Read the model definition and answer for the solid it produces. Units are mm, in the model's axes. A direction names the side the tool comes from. Give positions to 0.01 mm unless a question says otherwise; leave off trailing zeros. Loops run counter-clockwise (first coordinate to the right, second up) from the corner with the lowest first, then second, coordinate; pieces in that order, holes last. Notation, with made-up numbers: (76.5, 19) -> (98.5, 19) arc R10 ccw to (98.5, 27) -> close; hole circle Ø3 at (84.25, -34). An arc over 180 degrees is marked (long way). Return JSON: item names as keys, results as strings. Group by question number.
from build123d import *

# Parameters (mm, degrees)
EXTRUDE_2_DEPTH     = 2
CUT_EXTRUDE_2_DEPTH = 0.8
FILLET_1_R          = 0.8
SKETCH_6_W          = 43
SKETCH_6_H          = 2
SKETCH_6_H_2        = 1.9999999999999947
EXTRUDE_3_DEPTH     = 4
SKETCH_7_W          = 43
SKETCH_7_H          = 6.999999999999998
EXTRUDE_4_DEPTH     = 2
CUT_EXTRUDE_3_DEPTH = 35.3874977280988
CUT_EXTRUDE_5_DEPTH = 6
FILLET_2_R          = 4
FILLET_3_R          = 4
FILLET_4_R          = 4


# Some blends are built 0.0001 mm under size
with BuildPart() as part:
    # 草图4 → 凸台-拉伸2 (new body)
    with BuildSketch(Plane(origin=(0, 0, 0), x_dir=(1, 0, 0), z_dir=(0, 1, 0))):
        Polygon((24.499999999999996, -12.499999999999993), (24.499999999999996, 10.5), (24.499999999999996, 12.5), (-24.500000000000004, 12.5), (-28.500000000000004, 12.5), (-28.500000000000004, -12.499999999999993), (-24.500000000000004, -12.499999999999993), align=None)
        Polygon((-20.500000000000004, 10.500000000000002), (20.499999999999996, 10.5), (20.500000000000004, -10.5), (-20.5, -10.499999999999998), align=None, mode=Mode.SUBTRACT)
    extrude(amount=EXTRUDE_2_DEPTH)

    # 草图5 → 切除-拉伸2 (cut)
    with BuildSketch(Plane(origin=(0, 2, 0), x_dir=(1, 0, 0), z_dir=(0, 1, 0))):
        with BuildLine():
            Line((-24.000000000000004, 1.7499999999999991), (-24.000000000000004, 4.75))
            Line((-24.000000000000004, 4.75), (-21.000000000000004, 4.75))
            ThreePointArc((-21.000000000000004, 4.75), (-26.121320343559606, 6.871320343559683), (-24.000000000000117, 1.7499999999999991))
        make_face()
        with BuildLine():
            Line((-21.000000000000004, 4.75), (-24.000000000000004, 4.75))
            Line((-24.000000000000004, 4.75), (-24.000000000000004, 1.7499999999999991))
            ThreePointArc((-24.000000000000117, 1.7499999999999991), (-21.8786796564404, 2.6286796564403168), (-21.000000000000004, 4.749999999999999))
        make_face()
        with BuildLine():
            ThreePointArc((-21.000000000000007, -4.75), (-21.8786796564404, -2.6286796564403203), (-24.000000000000114, -1.7500000000000027))
            Line((-24.000000000000004, -1.7500000000000027), (-24.000000000000004, -4.75))
            Line((-24.000000000000004, -4.75), (-21.000000000000007, -4.75))
        make_face()
        with BuildLine():
            Line((-24.000000000000004, -4.75), (-24.000000000000004, -1.7500000000000027))
            ThreePointArc((-24.000000000000114, -1.7500000000000027), (-26.121320343559606, -6.871320343559679), (-21.000000000000007, -4.750000000000001))
            Line((-21.000000000000007, -4.75), (-24.000000000000004, -4.75))
        make_face()
        with BuildLine():
            Line((23.999999999999996, 4.75), (20.999999999999996, 4.75))
            ThreePointArc((21, 4.75), (21.878679656440315, 2.628679656440399), (23.999999999999883, 1.7500000000000027))
            Line((23.999999999999996, 1.7500000000000027), (23.999999999999996, 4.75))
        make_face()
        with BuildLine():
            ThreePointArc((24.50000000000003, 7.7080398915498), (22.063508326896304, 7.041287847477928), (21, 4.75))
            Line((20.999999999999996, 4.75), (23.999999999999996, 4.75))
            Line((23.999999999999996, 4.75), (23.999999999999996, 1.7500000000000027))
            ThreePointArc((23.999999999999883, 1.7500000000000027), (24.250878780839006, 1.760508431635119), (24.500000000000025, 1.7919601084501995))
            Line((24.499999999999996, 1.7919601084502048), (24.499999999999996, 7.708039891549795))
        make_face()
        with BuildLine():
            ThreePointArc((24.500000000000025, -1.7919601084501955), (24.25087878083901, -1.7605084316351154), (23.99999999999989, -1.7499999999999991))
            Line((24, -1.7499999999999991), (24, -4.75))
            Line((23.999999999999996, -4.75), (20.999999999999996, -4.75))
            ThreePointArc((21, -4.75), (22.0635083268963, -7.041287847477928), (24.50000000000002, -7.708039891549806))
            Line((24.499999999999996, -7.7080398915498005), (24.499999999999996, -1.7919601084501995))
        make_face()
        with BuildLine():
            Line((24, -4.75), (24, -1.7499999999999991))
            ThreePointArc((23.99999999999989, -1.7499999999999991), (21.87867965644032, -2.6286796564403963), (21, -4.75))
            Line((20.999999999999996, -4.75), (23.999999999999996, -4.75))
        make_face()
    extrude(amount=-CUT_EXTRUDE_2_DEPTH, mode=Mode.SUBTRACT)

    # 圆角1
    fillet_1_edges = [part.edges().sort_by_distance(p)[0] for p in [
        (21.000000000000117, 1.2, 4.749999999999868),
        (21, 1.2, -4.75),
        (-26.999999999999993, 1.2, 4.749999999999993),
        (-23.99999999999989, 1.2, -7.749999999999999),
    ]]
    fillet(fillet_1_edges, radius=FILLET_1_R - 0.0001)  # a hair under: the kernel refuses the full size

    # 草图6 → 凸台-拉伸3 (add)
    with BuildSketch(Plane(origin=(0, 2, 0), x_dir=(1, 0, 0), z_dir=(0, 1, 0))):
        with Locations((0.9999999999999947, 11.500000000000002)):
            Rectangle(SKETCH_6_W, SKETCH_6_H)
        with Locations((0.9999999999999982, -11.499999999999996)):
            Rectangle(SKETCH_6_W, SKETCH_6_H_2)
    extrude(amount=EXTRUDE_3_DEPTH)

    # 草图7 → 凸台-拉伸4 (add)
    with BuildSketch(Plane(origin=(0, 6, 0), x_dir=(1, 0, 0), z_dir=(0, 1, 0))):
        with Locations((0.9999999999999947, 14)):
            Rectangle(SKETCH_7_W, SKETCH_7_H)
        with Locations((0.9999999999999982, -13.999999999999996)):
            Rectangle(SKETCH_7_W, SKETCH_7_H)
    extrude(amount=EXTRUDE_4_DEPTH)

    # 草图8 → 切除-拉伸3 (cut, through all)
    with BuildSketch(Plane.XZ):
        with BuildLine():
            ThreePointArc((-10.5, -11.54), (-12.5, -13.54), (-10.5, -15.54))
            Line((-10.5, -15.54), (-6.500000000000001, -15.54))
            ThreePointArc((-6.500000000000001, -15.54), (-4.500000000000001, -13.54), (-6.500000000000001, -11.54))
            Line((-6.500000000000001, -11.54), (-10.5, -11.54))
        make_face()
        with BuildLine():
            ThreePointArc((14.5, -11.54), (12.5, -13.54), (14.5, -15.54))
            Line((14.5, -15.54), (18.500000000000004, -15.54))
            ThreePointArc((18.500000000000004, -15.54), (20.500000000000004, -13.54), (18.500000000000004, -11.54))
            Line((18.500000000000004, -11.54), (14.5, -11.54))
        make_face()
        with BuildLine():
            Line((-10.500000000000096, 11.54), (-6.500000000000095, 11.54))
            ThreePointArc((-6.500000000000095, 11.54), (-4.500000000000095, 13.54), (-6.500000000000095, 15.54))
            Line((-6.500000000000095, 15.54), (-10.500000000000096, 15.54))
            ThreePointArc((-10.500000000000096, 15.54), (-12.500000000000096, 13.54), (-10.500000000000096, 11.54))
        make_face()
        with BuildLine():
            Line((14.499999999999908, 11.54), (18.499999999999904, 11.54))
            ThreePointArc((18.499999999999904, 11.540000000000001), (20.499999999999904, 13.540000000000001), (18.499999999999904, 15.540000000000001))
            Line((18.499999999999904, 15.54), (14.499999999999908, 15.54))
            ThreePointArc((14.499999999999908, 15.54), (12.499999999999908, 13.54), (14.499999999999908, 11.54))
        make_face()
    extrude(amount=-CUT_EXTRUDE_3_DEPTH, mode=Mode.SUBTRACT)

    # 草图9 → 切除-拉伸5 (cut)
    with BuildSketch(Plane.XZ):
        with BuildLine():
            Line((14.5, -10.540000000000001), (18.500000000000004, -10.54))
            ThreePointArc((18.500000000000004, -10.54), (21.500000000000004, -13.54), (18.500000000000004, -16.54))
            Line((18.500000000000004, -16.54), (14.5, -16.54))
            ThreePointArc((14.5, -16.54), (11.500000000000002, -13.54), (14.5, -10.540000000000001))
        make_face()
        with BuildLine():
            Line((-10.5, -10.540000000000177), (-6.499999999999999, -10.540000000000175))
            ThreePointArc((-6.499999999999999, -10.540000000000175), (-3.500000000000001, -13.540000000000175), (-6.499999999999999, -16.540000000000173))
            Line((-6.499999999999999, -16.540000000000173), (-10.5, -16.540000000000173))
            ThreePointArc((-10.5, -16.540000000000173), (-13.499999999999998, -13.540000000000175), (-10.5, -10.540000000000177))
        make_face()
        with BuildLine():
            Line((-10.500000000000094, 16.539999999999825), (-6.500000000000092, 16.539999999999825))
            ThreePointArc((-6.500000000000092, 16.539999999999825), (-3.5000000000000924, 13.539999999999827), (-6.500000000000092, 10.539999999999827))
            Line((-6.500000000000092, 10.539999999999827), (-10.500000000000094, 10.539999999999827))
            ThreePointArc((-10.500000000000094, 10.539999999999827), (-13.500000000000092, 13.539999999999827), (-10.500000000000094, 16.539999999999825))
        make_face()
        with BuildLine():
            Line((14.499999999999906, 16.54), (18.499999999999908, 16.54))
            ThreePointArc((18.499999999999908, 16.54), (21.499999999999908, 13.54), (18.499999999999908, 10.540000000000001))
            Line((18.499999999999908, 10.540000000000001), (14.499999999999906, 10.540000000000001))
            ThreePointArc((14.499999999999906, 10.540000000000001), (11.499999999999906, 13.54), (14.499999999999906, 16.54))
        make_face()
    extrude(amount=-CUT_EXTRUDE_5_DEPTH, mode=Mode.SUBTRACT)

    # 圆角2
    # the kernel refuses this fillet: 4 mm, written as the material it takes off along each edge
    with BuildSketch(Plane(origin=(24.499999999999996, -9.790767556640994, 12.499999999999993), x_dir=(0, 0, -1), z_dir=(0, 1, 0))) as fillet_2_piece_1_section:
        with BuildLine():
            CenterArc((3.9163070226563974, 4), FILLET_2_R, 191.74119504503736, 78.25880495496267)
            Line((6.39666e-12, 3.186034826087571), (0, 0))
            Line((0, 0), (3.9163070226563974, 0))
        make_face()
    fillet_2_piece_1 = extrude(amount=21.581535113281987, mode=Mode.PRIVATE)
    fillet_2_piece_1 = split(fillet_2_piece_1, bisect_by=Plane(origin=(23.971029818368024, 6, 10.5876929773436), z_dir=(0, -1, 0)), keep=Keep.TOP, mode=Mode.PRIVATE)
    add(fillet_2_piece_1, mode=Mode.SUBTRACT)
    with BuildSketch(Plane(origin=(24.499999999999996, -9.790767556640994, -12.5), x_dir=(0, 0, 1), z_dir=(0, 1, 0))) as fillet_2_piece_2_section:
        with BuildLine():
            CenterArc((3.9163070226563974, -4), FILLET_2_R, 90, 78.25880495496122)
            Line((6.4162e-12, -3.186034826087475), (0, 0))
            Line((0, 0), (3.9163070226563974, 0))
        make_face()
    fillet_2_piece_2 = extrude(amount=21.581535113281987, mode=Mode.PRIVATE)
    fillet_2_piece_2 = split(fillet_2_piece_2, bisect_by=Plane(origin=(23.97102981836802, 6, -10.58769297734361), z_dir=(0, -1, 0)), keep=Keep.TOP, mode=Mode.PRIVATE)
    add(fillet_2_piece_2, mode=Mode.SUBTRACT)
    with BuildSketch(Plane(origin=(22.499999999999993, -4, -17.5), x_dir=(-1, 0, 0), z_dir=(0, 1, 0))) as fillet_2_piece_3:
        with BuildLine():
            CenterArc((FILLET_2_R, FILLET_2_R), FILLET_2_R, 180, 90)
            Line((0, FILLET_2_R), (0, 0))
            Line((0, 0), (FILLET_2_R, 0))
        make_face()
    extrude(amount=22, mode=Mode.SUBTRACT)
    with BuildSketch(Plane(origin=(22.499999999999996, -4, 17.499999999999996), x_dir=(-1, 0, 0), z_dir=(0, 1, 0))) as fillet_2_piece_4:
        with BuildLine():
            CenterArc((FILLET_2_R, -FILLET_2_R), FILLET_2_R, 90, 90)
            Line((0, -FILLET_2_R), (0, 0))
            Line((0, 0), (FILLET_2_R, 0))
        make_face()
    extrude(amount=22, mode=Mode.SUBTRACT)

    # 圆角3
    fillet_3_edges = [part.edges().sort_by_distance(p)[0] for p in [
        (-28.500000000000004, 1, 12.499999999999993),
        (-28.500000000000004, 1, -12.5),
    ]]
    fillet(fillet_3_edges, radius=FILLET_3_R)

    # 圆角4
    fillet_4_edges = [part.edges().sort_by_distance(p)[0] for p in [
        (-20.5, 7, 17.499999999999996),
        (-20.500000000000004, 7, -17.5),
    ]]
    fillet(fillet_4_edges, radius=FILLET_4_R)


solid = part.part
1. Determine the mould class of faces 1 (the cylindrical face through (23.214, 1.625, -11.522)), 2 (the flat face through (1, 7, 17.5)), 3 (the flat face through (-8, 7, -11.54)), 4 (the cylindrical face through (-12.5, 7, 13.6)) for opening direction Z: pulls with the +Z half, pulls with the -Z half, needs draft (parallel to the pull), parting line crosses it, or undercut.
2. Which of the six approach directions +Z, -Z, +X, -X, +Y, -Y give full straight-line access (tool end or side, diameter ignored) to faces 5 (the cylindrical face through (12.764, 2.958, -11.093)), 6 (the flat face through (-24, 1.2, -5)), 7 (the cylindrical face through (-4.5, 7, -13.6)), 8 (the flat face through (23, 1.2, 5)), 9 (the cylindrical face through (20.236, 2.958, 11.093))?
3. Section A-A on y = 5 is taken. Determine the outline of the cut face in (x, z), then the cut area to 3 significant figures.
4. Flat-ended cylindrical pins translate along their axes: pin 1 Ø3 at (x, y) = (2.5, 3) entering from -Z; pin 2 Ø3.5 at (x, z) = (1.5, 15.5) entering from -Y; pin 3 Ø3.5 at (y, z) = (5.5, 12.5) entering from -X. Find the tip coordinate at first contact, or state that the pin passes through.
5. Section D-D on z = 15 is taken. Determine the outline of the cut face in (x, y).
6. Section C-C on x = 17 is taken. State how many separate pieces and enclosed holes the cut face has, then the cut area to 3 significant figures.
7. Straight lines are drawn through the part: line 1 (X direction, y = 6.5, z = 14); line 2 (Z direction, x = 1.5, y = 7.5); line 3 (Z direction, x = 2.5, y = 3.25). For each, find the intervals that lie inside material, in ascending order. Write a range as from..to.
Completed:
{
 "1": {"face 1": "pulls with the -Z half", "face 2": "pulls with the +Z half", "face 3": "undercut", "face 4": "undercut"},
 "2": {"face 5": "-Z, -Y", "face 6": "+Y", "face 7": "+Y, -Y", "face 8": "+X, +Y", "face 9": "+Z, -Y"},
 "3": {"outline": "(-20.5, -12.5) -> (-13.31, -12.5) arc R3 cw to (-10.5, -10.54) -> (-6.5, -10.54) arc R3 cw to (-3.69, -12.5) -> (11.69, -12.5) arc R3 cw to (14.5, -10.54) -> (18.5, -10.54) arc R3 cw to (21.31, -12.5) arc R4 ccw to (22.5, -12.05) -> (22.5, -10.5) -> (-20.5, -10.5) -> close; (-20.5, 10.5) -> (22.5, 10.5) -> (22.5, 12.05) arc R4 ccw to (21.31, 12.5) arc R3 cw to (18.5, 10.54) -> (14.5, 10.54) arc R3 cw to (11.69, 12.5) -> (-3.69, 12.5) arc R3 cw to (-6.5, 10.54) -> (-10.5, 10.54) arc R3 cw to (-13.31, 12.5) -> (-20.5, 12.5) -> close", "area": "108 mm²"},
 "4": {"pin 1": "stops at z = -12.5", "pin 2": "stops at y = 6", "pin 3": "stops at x = -20.5"},
 "5": {"outline": "(-20.21, 6) -> (-11.87, 6) -> (-11.87, 8) -> (-20.21, 8) -> close; (-5.13, 6) -> (13.13, 6) -> (13.13, 8) -> (-5.13, 8) -> close; (19.87, 6) -> (22.21, 6) -> (22.21, 8) -> (19.87, 8) -> close"},
 "6": {"separate pieces": "4", "enclosed holes": "0", "area": "12.5 mm²"},
 "7": {"line 1": "x = -20.47..-12.45, -4.55..12.55, 20.45..22.47", "line 2": "z = -17.5..-10.5, 10.5..17.5", "line 3": "z = -12.5..-10.5, 10.5..12.5"}
}
